Read the model definition and answer for the solid it produces. Units are mm, in the model's axes. A direction names the side the tool comes from. Give positions to 0.01 mm unless a question says otherwise; leave off trailing zeros. Order: outer loops, then holes, each group sorted by start corner. A loop starts at its lowest first (then second) coordinate and runs counter-clockwise, first axis right, second up. Notation, with made-up numbers: (43, 58) - (85, 58) arc R25 ccw to (85, 87) - close; hole circle Ø9 at (66, 39). An arc over 180 degrees is marked (long way). Write item = value, one per line.
```python
from build123d import *

# Parameters (mm, degrees)
SKETCH_1_W          = 180
SKETCH_1_H          = 110
EXTRUDE_1_DEPTH     = 30
SKETCH_2_W          = 150
SKETCH_2_H          = 75
CUT_EXTRUDE_1_DEPTH = 30
SKETCH_3_W          = 20
SKETCH_3_H          = 40
CUT_EXTRUDE_2_DEPTH = 150
SKETCH_4_W          = 20
SKETCH_4_H          = 80
CUT_EXTRUDE_3_DEPTH = 30
SKETCH_5_W          = 120
SKETCH_5_H          = 22
CUT_EXTRUDE_4_DEPTH = 30
SKETCH_6_W          = 100
SKETCH_6_H          = 10
CUT_EXTRUDE_5_DEPTH = 64
EXTRUDE_2_DEPTH     = 10
EXTRUDE_3_DEPTH     = 10
SKETCH_9_W          = 180
SKETCH_9_H          = 50
EXTRUDE_4_DEPTH     = 15
SKETCH_10_R         = 5
CUT_EXTRUDE_6_DEPTH = 144
SKETCH_11_R         = 7.5
CUT_EXTRUDE_7_DEPTH = 191


with BuildPart() as part:
    # 草图1 → 凸台-拉伸1 (new body)
    with BuildSketch(Plane.XY):
        Rectangle(SKETCH_1_W, SKETCH_1_H)
    extrude(amount=EXTRUDE_1_DEPTH)

    # 草图2 → 切除-拉伸1 (cut)
    with BuildSketch(Plane.XY.offset(30)):
        with Locations((-15, -17.5)):
            Rectangle(SKETCH_2_W, SKETCH_2_H)
    extrude(amount=-CUT_EXTRUDE_1_DEPTH, mode=Mode.SUBTRACT)

    # 草图3 → 切除-拉伸2 (cut)
    with BuildSketch(Plane.ZY.offset(90)):
        with Locations((15, 20)):
            Rectangle(SKETCH_3_W, SKETCH_3_H)
    extrude(amount=-CUT_EXTRUDE_2_DEPTH, mode=Mode.SUBTRACT)

    # 草图4 → 切除-拉伸3 (cut)
    with BuildSketch(Plane.ZY.offset(-60)):
        with Locations((15, -55)):
            Rectangle(SKETCH_4_W, SKETCH_4_H)
    extrude(amount=-CUT_EXTRUDE_3_DEPTH, mode=Mode.SUBTRACT)

    # 草图5 → 切除-拉伸4 (cut)
    with BuildSketch(Plane.XY.offset(30)):
        with Locations((0, 31)):
            Rectangle(SKETCH_5_W, SKETCH_5_H)
    extrude(amount=-CUT_EXTRUDE_4_DEPTH, mode=Mode.SUBTRACT)

    # 草图6 → 切除-拉伸5 (cut)
    with BuildSketch(Plane.XZ.offset(15)):
        with Locations((0, 15)):
            Rectangle(SKETCH_6_W, SKETCH_6_H)
    extrude(amount=-CUT_EXTRUDE_5_DEPTH, mode=Mode.SUBTRACT)

    # 草图7 → 凸台-拉伸2 (add)
    with BuildSketch(Plane(origin=(0, 0, 0), x_dir=(-1, 0, 0), z_dir=(0, 0, -1))):
        Polygon((-60, 42), (60, 42), (60, 20), (90, 20), (90, 55), (-90, 55), (-90, -55), (-60, -55), align=None)
    extrude(amount=EXTRUDE_2_DEPTH)

    # 草图8 → 凸台-拉伸3 (add)
    with BuildSketch(Plane.XY.offset(30)):
        Polygon((-60, 20), (-60, 42), (60, 42), (60, -55), (90, -55), (90, 55), (-90, 55), (-90, 20), align=None)
    extrude(amount=EXTRUDE_3_DEPTH)

    # 草图9 → 凸台-拉伸4 (add)
    with BuildSketch(Plane(origin=(0, 55, 0), x_dir=(1, 0, 0), z_dir=(0, 1, 0))):
        with Locations((0, -15)):
            Rectangle(SKETCH_9_W, SKETCH_9_H)
    extrude(amount=EXTRUDE_4_DEPTH)

    # 草图10 → 切除-拉伸6 (cut)
    with BuildSketch(Plane.XZ.offset(55)):
        with Locations((75, 40)):
            Circle(SKETCH_10_R)
        with Locations((75, -10)):
            Circle(SKETCH_10_R)
        with Locations((-75, 40)):
            Circle(SKETCH_10_R)
        with Locations((-75, -10)):
            Circle(SKETCH_10_R)
    extrude(amount=-CUT_EXTRUDE_6_DEPTH, mode=Mode.SUBTRACT)

    # 草图11 → 切除-拉伸7 (cut)
    with BuildSketch(Plane.ZY.offset(90)):
        with Locations((40, 55)):
            Circle(SKETCH_11_R)
        with Locations((-10, 55)):
            Circle(SKETCH_11_R)
    extrude(amount=-CUT_EXTRUDE_7_DEPTH, mode=Mode.SUBTRACT)


solid = part.part
```
1. Section B-B (z = 7) is taken. Determine the outline of the cut face in (x, y).
Recorded:
outline = (-90, 40) - (-60, 40) - (-60, 42) - (60, 42) - (60, -15) - (90, -15) - (90, 70) - (-90, 70) - close
2. Straight lines are drawn through the part: L1, parallel to Z at x = -81, y = 35; L2, parallel to X at y = 16, z = 34.5; L3, parallel to Y at x = -46, z = 32. For each, find the intervals that lie inside material, in ascending order. Write a range as [from, to].
Recorded:
L1 = [-10, 5], [25, 40]
L2 = [60, 90]
L3 = [42, 70]
3. Section A-A (y = -37) is taken. Determine the outline of the cut face in (x, z).
Recorded:
outline = (60, -10) - (70, -10) arc R5 cw to (80, -10) - (90, -10) - (90, 5) - (60, 5) - close; (60, 25) - (90, 25) - (90, 40) - (80, 40) arc R5 cw to (70, 40) - (60, 40) - close
4. Section D-D (x = -47) is taken. Determine the outline of the cut face in (y, z).
Recorded:
outline = (42, -10) - (47.5, -10) arc R7.5 cw to (62.5, -10) - (70, -10) - (70, 40) - (62.5, 40) arc R7.5 cw to (47.5, 40) - (42, 40) - (42, 20) - (49, 20) - (49, 10) - (42, 10) - close
5. Flat-ended cylindrical pins translate along their axes: pin 1 (4 mm diameter, centred on x = -47.5, y = 53, fed in from +Z); pin 2 (16 mm diameter, centred on x = -73.5, y = 25.5, fed in from +Z); pin 3 (4.5 mm diameter, centred on x = -82, z = 0.5, fed in from -Y); pin 4 (6 mm diameter, centred on x = -77, z = 14.5, fed in from -Y). Find the tip coordinate at first contact, or state that the pin passes through.
Recorded:
pin_1 = 33.66
pin_2 = 40
pin_3 = 20
pin_4 = 40
6. For faces 1 (the face through (-50, 45, 15)), 2 (the face through (75, -35, 25)), 3 (the face through (-75, 30, 5)), determine the directions among +Z, -Z, +X, -X, +Y, -Y from which every point of the face is accessible in a straight line to the end or side of a thin tool.
Recorded:
face_1 = -Y
face_2 = +X, -X, -Y
face_3 = -X, -Y
7. Section C-C (x = -75) is taken. Determine the outline of the cut face in (y, z).
Recorded:
outline = (20, -5) - (49.41, -5) arc R7.5 cw to (60.59, -5) - (70, -5) - (70, 35) - (60.59, 35) arc R7.5 cw to (49.41, 35) - (20, 35) - (20, 25) - (40, 25) - (40, 5) - (20, 5) - close
8. Determine the mould class of faces 4 (the face through (-75, 34, -5)), 5 (the face through (-1, 49, 15)), 6 (the face through (-90, 45, 15)) for opening direction Z: +Z half, -Z half, draft (parallel to the pull), parting line (faces both ways), or undercut.
Recorded:
face_4 = -Z half
face_5 = undercut
face_6 = draft
